Input: part model. Units: mm. Frame: model coordinates. Face numbers are marked on the shaded views. Give positions to 0.01 mm unless a question says otherwise; leave off trailing zeros. Write each loop counter-clockwise with the first axis right and the second up, starting at its lowest first coordinate (ties: lowest second). Pieces come first, ordered by that corner, then holes.
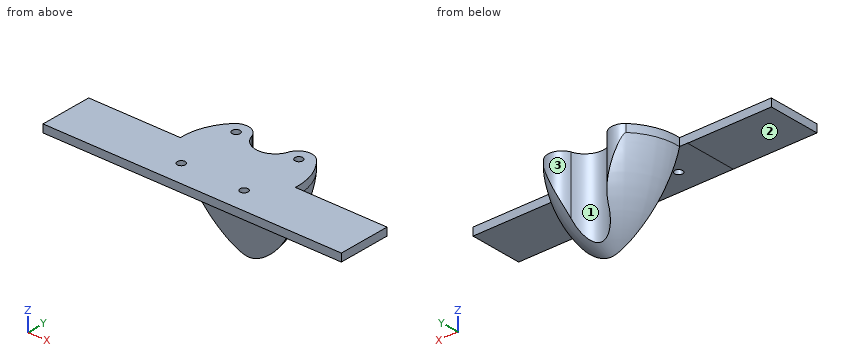
```python
from build123d import *

# Parameters (mm, degrees)
F0_R     = 1.5
F1_DEPTH = 3
F5_DEPTH = 25
F7_DEPTH = 35


# Not quite as in the source:
# - a feature names something its author has since deleted; it is built from what else it names


with BuildPart() as f1:
    # F0 (on Top) → F1 (new body)
    with BuildSketch(Plane.XY):
        with BuildLine():
            Line((6.5574385243, -21), (57, -21))
            Line((57, -21), (57, -1))
            Line((57, -1), (21.9772609758, -1))
            ThreePointArc((21.9772609758, -1), (0, 22), (-21.9772609758, -1))
            Line((-21.9772609758, -1), (-57, -1))
            Line((-57, -1), (-57, -21))
            Line((-57, -21), (6.5574385243, -21))
        make_face()
        with Locations((-12, -12)):
            Circle(F0_R, mode=Mode.SUBTRACT)
        with Locations((12, -12)):
            Circle(F0_R, mode=Mode.SUBTRACT)
        with Locations((-12, 12)):
            Circle(F0_R, mode=Mode.SUBTRACT)
        with Locations((12, 12)):
            Circle(F0_R, mode=Mode.SUBTRACT)
    extrude(amount=F1_DEPTH)

    # F2 (on Right) → F3 (revolve)
    with BuildSketch(Plane.YZ):
        with BuildLine():
            Line((0, 0), (0, -32.8796606992))
            ThreePointArc((0, -32.8796606992), (15.0334447446, -19.1386350968), (22, 0))
            Line((22, 0), (0, 0))
        make_face()
    revolve(axis=Axis((0, 0, -16.4398303496), (0, 0, -1)))

    # F4 (on Right) → F5 (cut, symmetric)
    with BuildSketch(Plane.YZ):
        Polygon((7.20365692, -51.6230810942), (-0.9809204616, 0.0523067461), (-22.7521642769, 0), (-21.7191129923, -52.1955192089), align=None)
    extrude(amount=F5_DEPTH, both=True, mode=Mode.SUBTRACT)

    # F6 (on face) → F7 (cut)
    with BuildSketch(Plane.XY.offset(3)):
        with BuildLine():
            ThreePointArc((-15.7890972634, 15.3200655223), (-10.8662470151, 16.6578455627), (-7.0613301317, 13.2597994308))
            ThreePointArc((-7.0613301317, 13.2597994308), (0, 8.0029264883), (7.0613301317, 13.2597994308))
            ThreePointArc((7.0613301317, 13.2597994308), (10.8662470151, 16.6578455627), (15.7890972634, 15.3200655223))
            ThreePointArc((15.7890972634, 15.3200655223), (0, 22), (-15.7890972634, 15.3200655223))
        make_face()
    extrude(amount=-F7_DEPTH, mode=Mode.SUBTRACT)


solid = f1.part
```
Item 1: Section B-B (x = 34). Return loops of the section in (y, z).
Item 2: Pin query (flat end, axial travel): pin 1 (4 mm diameter, centred on x = 30, z = -0.5, fed in from +Y); pin 2 (5 mm diameter, centred on x = -32.5, y = -5, fed in from -Z); pin 3 (2.5 mm diameter, centred on x = -12, y = 12, fed in from -Z). Return the tip coordinate at first contact, or that it passes through.
Item 3: Ray query, line 1 (X direction, y = -12, z = 1.2); line 2 (Y direction, x = -12, z = 1.55); line 3 (Z direction, x = -5, y = -9.5). Return the intervals inside material, ascending.
Item 4: Mould query, pull axis X, two halves, no side actions, for the marked faces 1, 2 and 3. Classes: +X half, -X half, draft (parallel to the pull), parting line (faces both ways), or undercut.
Item 5: Section A-A (y = -12). Give the number of separate pieces and of enclosed holes in the cut face, and give its area (3 significant figures).
Solved:
1. outline: (-21, 0) - (-1, 0) - (-1, 3) - (-21, 3) - close
2. pin 1: stops at y = -1
2. pin 2: stops at z = 0
2. pin 3: stops at z = -18.08
3. line 1: x = -57 to -13.5, -10.5 to 10.5, 13.5 to 57
3. line 2: y = -21 to -13.5, -10.5 to 10.5, 13.5 to 16.8
3. line 3: z = 0.03 to 3
4. face 1: undercut
4. face 2: draft
4. face 3: undercut
5. separate pieces: 3
5. enclosed holes: 0
5. area: 323 mm2
